from build123d import *

# Parameters (mm, degrees)
SKETCH2_W           = 20
SKETCH2_H           = 50
BOSS_EXTRUDE1_DEPTH = 44.5
SKETCH3_W           = 6.8
SKETCH3_H           = 21.48
SKETCH3_W_2         = 5
SKETCH3_H_2         = 15.77
CUT_EXTRUDE3_DEPTH  = 68.677544282
SKETCH4_R           = 3
CUT_EXTRUDE4_DEPTH  = 55.820160525
SKETCH4_3_R         = 3
SKETCH4_3_R_2       = 2.1
CUT_EXTRUDE5_DEPTH  = 6.6
BOSS_EXTRUDE2_START = -6.6
SKETCH5_R           = 3
SKETCH5_R_2         = 2.6
BOSS_EXTRUDE2_DEPTH = 6.6
SKETCH6_R           = 3.1
CUT_EXTRUDE6_DEPTH  = 1.23
SKETCH8_R           = 3.35
CUT_EXTRUDE8_DEPTH  = 0.8
CIRPATTERN1_COUNT   = 2
CIRPATTERN1_ANGLE   = 180
SKETCH12_R          = 2.35
CUT_EXTRUDE9_DEPTH  = 6.6


with BuildPart() as part:
    # Sketch2 → Boss-Extrude1 (new body)
    with BuildSketch(Plane(origin=(0, 0, 0), x_dir=(1, 0, 0), z_dir=(0, 1, 0))):
        Rectangle(SKETCH2_W, SKETCH2_H)
    extrude(amount=BOSS_EXTRUDE1_DEPTH)

    # Sketch3 → Cut-Extrude3 (cut, through all)
    with BuildSketch(Plane.XY.offset(25)):
        with Locations((0, 33.76)):
            Rectangle(SKETCH3_W, SKETCH3_H)
        with Locations((0, 15.135)):
            Rectangle(SKETCH3_W_2, SKETCH3_H_2)
    extrude(amount=-CUT_EXTRUDE3_DEPTH, mode=Mode.SUBTRACT)

    # Sketch4 → Cut-Extrude4 (cut, through all)
    with BuildSketch(Plane(origin=(10, 0, 0), x_dir=(0, 0, -1), z_dir=(1, 0, 0))):
        with Locations((-13, 32.41)):
            Circle(SKETCH4_R)
    cut_extrude4 = extrude(amount=-CUT_EXTRUDE4_DEPTH, mode=Mode.SUBTRACT)

    # Sketch4_3 → Cut-Extrude5 (cut)
    with BuildSketch(Plane(origin=(10, 0, 0), x_dir=(0, 0, -1), z_dir=(1, 0, 0))):
        with Locations((-13, 32.41)):
            Circle(SKETCH4_3_R)
        with Locations((-13, 19.71)):
            Circle(SKETCH4_3_R_2)
        with Locations((-6.65, 38.76)):
            Circle(SKETCH4_3_R_2)
        with Locations((-6.65, 26.06)):
            Circle(SKETCH4_3_R_2)
        with Locations((-6.65, 13.36)):
            Circle(SKETCH4_3_R_2)
        with Locations(Location((-19.35, 13.36, 0), (0, 0, 180))):
            Circle(SKETCH4_3_R_2)
        with Locations(Location((-19.35, 26.06, 0), (0, 0, 180))):
            Circle(SKETCH4_3_R_2)
        with Locations(Location((-19.35, 38.76, 0), (0, 0, 180))):
            Circle(SKETCH4_3_R_2)
    cut_extrude5 = extrude(amount=-CUT_EXTRUDE5_DEPTH, mode=Mode.SUBTRACT)

    # Sketch5 → Boss-Extrude2 (add)
    with BuildSketch(Plane.ZY.offset(10).offset(BOSS_EXTRUDE2_START)):
        with Locations(Location((13, 32.41, 0), (0, 0, 180))):
            Circle(SKETCH5_R)
        with Locations((13, 32.41)):
            Circle(SKETCH5_R_2, mode=Mode.SUBTRACT)
    boss_extrude2 = extrude(amount=BOSS_EXTRUDE2_DEPTH)

    # Sketch6 → Cut-Extrude6 (cut)
    with BuildSketch(Plane.ZY.offset(-3.4)):
        with Locations(Location((6.65, 13.36, 0), (0, 0, 270))):
            Circle(SKETCH6_R)
        with Locations(Location((6.65, 26.06, 0), (0, 0, 270))):
            Circle(SKETCH6_R)
        with Locations(Location((13, 19.71, 0), (0, 0, 270))):
            Circle(SKETCH6_R)
        with Locations(Location((19.35, 13.36, 0), (0, 0, 270))):
            Circle(SKETCH6_R)
        with Locations(Location((19.35, 26.06, 0), (0, 0, 270))):
            Circle(SKETCH6_R)
        with Locations(Location((19.35, 38.76, 0), (0, 0, 270))):
            Circle(SKETCH6_R)
        with Locations(Location((6.65, 38.76, 0), (0, 0, 270))):
            Circle(SKETCH6_R)
    cut_extrude6 = extrude(amount=-CUT_EXTRUDE6_DEPTH, mode=Mode.SUBTRACT)

    # Sketch8 → Cut-Extrude8 (cut)
    with BuildSketch(Plane(origin=(10, 0, 0), x_dir=(0, 0, -1), z_dir=(1, 0, 0))):
        with Locations((-6.65, 38.76)):
            Circle(SKETCH8_R)
        with Locations((-6.65, 26.06)):
            Circle(SKETCH8_R)
        with Locations((-6.65, 13.36)):
            Circle(SKETCH8_R)
        with Locations((-13, 19.71)):
            Circle(SKETCH8_R)
        with Locations((-19.35, 38.76)):
            Circle(SKETCH8_R)
        with Locations((-19.35, 26.06)):
            Circle(SKETCH8_R)
        with Locations((-19.35, 13.36)):
            Circle(SKETCH8_R)
    cut_extrude8 = extrude(amount=-CUT_EXTRUDE8_DEPTH, mode=Mode.SUBTRACT)

    # CirPattern1: Cut-Extrude4, Cut-Extrude5, Boss-Extrude2, Cut-Extrude6, Cut-Extrude8 ×2 about axis
    cirpattern1_axis = Axis((0, 44.5, 0), (0, -1, 0))
    add([cut_extrude4.rotate(cirpattern1_axis, i * CIRPATTERN1_ANGLE / (CIRPATTERN1_COUNT - 1)) for i in range(1, CIRPATTERN1_COUNT)], mode=Mode.SUBTRACT)
    add([cut_extrude5.rotate(cirpattern1_axis, i * CIRPATTERN1_ANGLE / (CIRPATTERN1_COUNT - 1)) for i in range(1, CIRPATTERN1_COUNT)], mode=Mode.SUBTRACT)
    add([boss_extrude2.rotate(cirpattern1_axis, i * CIRPATTERN1_ANGLE / (CIRPATTERN1_COUNT - 1)) for i in range(1, CIRPATTERN1_COUNT)])
    add([cut_extrude6.rotate(cirpattern1_axis, i * CIRPATTERN1_ANGLE / (CIRPATTERN1_COUNT - 1)) for i in range(1, CIRPATTERN1_COUNT)], mode=Mode.SUBTRACT)
    add([cut_extrude8.rotate(cirpattern1_axis, i * CIRPATTERN1_ANGLE / (CIRPATTERN1_COUNT - 1)) for i in range(1, CIRPATTERN1_COUNT)], mode=Mode.SUBTRACT)

    # Sketch12 → Cut-Extrude9 (cut)
    with BuildSketch(Plane(origin=(-10, 0, 0), x_dir=(0, 0, -1), z_dir=(1, 0, 0))):
        with Locations((-13, 6.59)):
            Circle(SKETCH12_R)
    extrude(amount=CUT_EXTRUDE9_DEPTH, mode=Mode.SUBTRACT)


solid = part.part
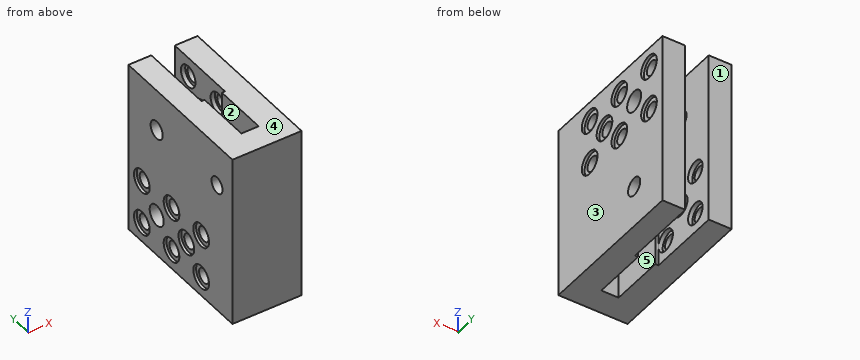
Work out the finished part from the listing and answer in its coordinate system (mm). Face numbers are marked on the shaded views. A direction names the side the tool comes from. Round coordinates to 2 decimals unless told otherwise and drop trailing zeros. Write each loop counter-clockwise with the first axis right and the second up, starting at its lowest first coordinate (ties: lowest second). Pieces come first, ordered by that corner, then holes. Notation, with made-up numbers: (7.25, 9.25) -> (48.25, 9.25) arc R16 cw to (48.25, 37.25) -> close; hole circle Ø1 at (40.5, -39). An arc over 180 degrees is marked (long way). Answer as CSV lines item,"result". Start each with the question number.
(1) The mould has two halves that part along X. Classify the marked faces 3, 4 and 5: +X half, -X half, draft (parallel to the pull), parting line (faces both ways), or undercut.
(2) Each of these flat-tipped pins is pushed along its axis until it touches: pin 1 (3.5 mm diameter, centred on y = 13, z = -6.5, fed in from -X); pin 2 (1.9 mm diameter, centred on y = 12, z = 7, fed in from +X). Where does it stop, or does it pass through?
(3) Find the intervals of material crossed by probe 1 along X at (y, z) = (11, -7.5); probe 2 along Y at (x, z) = (9.4, 6.65); probe 3 along Y at (x, z) = (6.1, 19.35), in increasing order.
(4) The part is cut by section B-B, the plane y = 32.41. Give the vertices of the cut face in (x, z), then the cut area to 3 significant figures.
(5) The part is cut by section A-A, the plane z = -13. Give the number of separate pieces and of enclosed holes in the cut face, then the cut area to 3 significant figures.
(6) A tool of negligible diameter and unlimited length cuts with its end or side. For the marked faces 1 and 2, from which of +Z, -Z, +X, -X, +Y, -Y can it reach the whole face along a straight path? Write none if from no direction.
Output values:
1,face 3,"+X half"
1,face 4,"draft"
1,face 5,"undercut"
2,pin 1,"stops at x = -9.2"
2,pin 2,"stops at x = 9.2"
3,probe 1,"x = -9.2 to -4.63, -3.4 to -2.5, 2.5 to 10"
3,probe 2,"y = 0 to 10.01, 16.71 to 22.71, 29.41 to 35.41, 42.11 to 44.5"
3,probe 3,"y = 0 to 11.26, 15.46 to 23.96, 28.16 to 36.66, 40.86 to 44.5"
4,outline,"(-10, -25) -> (-3.4, -25) -> (-3.4, -16) -> (-10, -16) -> close; (-10, -10) -> (-3.4, -10) -> (-3.4, 10.4) -> (-10, 10.4) -> close; (-10, 15.6) -> (-3.4, 15.6) -> (-3.4, 25) -> (-10, 25) -> close; (3.4, -25) -> (10, -25) -> (10, -15.6) -> (3.4, -15.6) -> close; (3.4, -10.4) -> (10, -10.4) -> (10, 10) -> (3.4, 10) -> close; (3.4, 16) -> (10, 16) -> (10, 25) -> (3.4, 25) -> close"
4,area,"512 mm²"
5,separate pieces,"3"
5,enclosed holes,"0"
5,area,"559 mm²"
6,face 1,"+Z, -Z, +X, -X, +Y"
6,face 2,"+Z, -Z, +Y"
